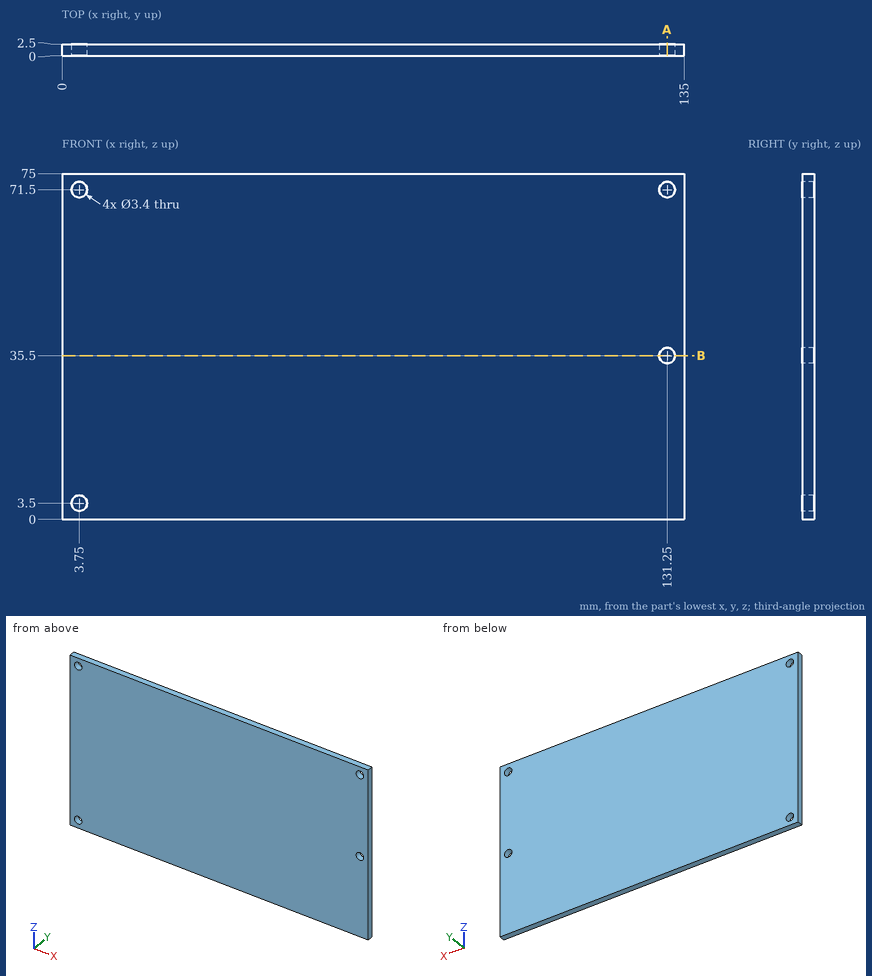
Design review of the part shown in the three views and the two pictorial views. Dimensions are in mm from the part's minimum x, y and z. Coordinates: 2 decimals unless noted, no trailing zeros. Order: outer loops, then holes, each group sorted by start corner. A loop starts at its lowest first (then second) coordinate and runs counter-clockwise, first axis right, second up.
Item 1: For pin 1 Ø4 at (x, z) = (131.25, 35.5) entering from +Y, flat-tipped, find the tip position at first contact; note if it passes through.
Item 2: Take a section at A-A, the plane x = 131.25. Write out the cut boundary in (y, z).
Item 3: Take a section at B-B, the plane z = 35.5. Write out the cut boundary in (x, y).
Item 4: For line 1 (Z direction, x = 131.25, y = 1.75); line 2 (Z direction, x = 3.75, y = 0.8); line 3 (X direction, y = 1.65, z = 71.5), list the stretches that pass through material, from the lowest coordinate up.
The answers:
1. pin 1: stops at y = 2.5
2. outline: (0, 0) - (2.5, 0) - (2.5, 33.8) - (0, 33.8) - close; (0, 37.2) - (2.5, 37.2) - (2.5, 69.8) - (0, 69.8) - close; (0, 73.2) - (2.5, 73.2) - (2.5, 75) - (0, 75) - close
3. outline: (0, 0) - (129.55, 0) - (129.55, 2.5) - (0, 2.5) - close; (132.95, 0) - (135, 0) - (135, 2.5) - (132.95, 2.5) - close
4. line 1: z = 0 to 33.8, 37.2 to 69.8, 73.2 to 75
4. line 2: z = 0 to 1.8, 5.2 to 69.8, 73.2 to 75
4. line 3: x = 0 to 2.05, 5.45 to 129.55, 132.95 to 135
